Verification items for the finished model (mm, model axes). A direction names the side the tool comes from. Coordinates: 2 decimals unless noted, no trailing zeros. Order: outer loops, then holes, each group sorted by start corner. A loop starts at its lowest first (then second) coordinate and runs counter-clockwise, first axis right, second up. Notation, with made-up numbers: (52, 12) -> (57, 12) arc R14 cw to (57, 36) -> close; hole circle Ø1 at (51.25, -37). An arc over 180 degrees is marked (long way). Use CSV: the item, a comma, the result in double quotes. Start each with the question number.
1) Scan lines: line 1 along Y through (x, z) = (0, -1.9); line 2 along Y through (x, z) = (0, -0.8). Record each from-to range of solid material in increasing order.
2) Tool access check on faces 1 (the flat face through (8.6, 16.4, -0.508)), 2 (the flat face through (2.76, 1.57, 1.54)), 3 (the cylindrical face through (-0.33, -2.52, -1.77)). Record the directions out of +Z, -Z, +X, -X, +Y, -Y that give a thin tool (end or side, any length) a straight path to the whole face; none if there is none.
3) Sectioned sample at B-B on x = 0. Record the boundary of the cut face in (y, z) (3 decimals), then the cut area to 3 significant figures.
4) Release check for a two-part mould opening along X. For faces 4 (the cylindrical face through (0.201, 38.098, 1.377)), 5 (the flat face through (0.1, 3.556, -0.5)), 6 (the flat face through (2.737, -1.61, 1.542)), 7 (the flat face through (0, 15, 2.794)) record: released by +X, released by -X, zero draft, split by the parting line, or undercut.
5) Sectioned sample at A-A on z = 2.35. Record the boundary of the cut face in (x, y) (3 decimals).
6) Go/stop test with flat-tipped pins: pin 1 (0.8 mm diameter, centred on x = -9, y = 11.5, fed in from -Z); pin 2 (4.5 mm diameter, centred on x = 0, y = 0, fed in from +Z); pin 3 (1 mm diameter, centred on x = -2, y = 29, fed in from -Z). Record where each tip stops, or that it passes through.
7) Sectioned sample at C-C on y = 8. Record the boundary of the cut face in (x, z).
8) Sectioned sample at D-D on x = 4.25. Record the boundary of the cut face in (y, z).
from build123d import *

# Parameters (mm, degrees)
F0_W     = 1.016
F0_H     = 3.556
F0_H_2   = 5.588
F1_DEPTH = 2.794
F2_DEPTH = 0.508
F3_DEPTH = 1.016
F4_R     = 2.54
F5_DEPTH = 1.524
F6_R     = 1.397
F7_DEPTH = 5.334
F9_DEPTH = 2.54


with BuildPart() as f1:
    # F0 (on Top) → F1 (new body)
    with BuildSketch(Plane.XY):
        with BuildLine():
            Line((8.128, 28.956), (9.144, 28.956))
            ThreePointArc((9.144, 28.956), (0, 38.1), (-9.144, 28.956))
            Line((-9.144, 28.956), (-8.128, 28.956))
            Line((-8.128, 28.956), (-2.54, 28.956))
            ThreePointArc((-2.54, 28.956), (0, 31.496), (2.54, 28.956))
            Line((2.54, 28.956), (8.128, 28.956))
        make_face()
        with BuildLine():
            ThreePointArc((-8.128, 24.7669246844), (0, 19.812), (8.128, 24.7669246844))
            Line((8.128, 24.7669246844), (8.128, 28.956))
            Line((8.128, 28.956), (2.54, 28.956))
            ThreePointArc((2.54, 28.956), (0, 26.416), (-2.54, 28.956))
            Line((-2.54, 28.956), (-8.128, 28.956))
            Line((-8.128, 28.956), (-8.128, 24.7669246844))
        make_face()
        with BuildLine():
            Line((8.128, 24.7669246844), (8.128, 9.144))
            Line((8.128, 9.144), (9.144, 9.144))
            Line((9.144, 9.144), (9.144, 28.956))
            ThreePointArc((9.144, 28.956), (8.8863706877, 26.8007385309), (8.128, 24.7669246844))
        make_face()
        with BuildLine():
            Line((8.128, 28.956), (8.128, 24.7669246844))
            ThreePointArc((8.128, 24.7669246844), (8.8863706877, 26.8007385309), (9.144, 28.956))
            Line((9.144, 28.956), (8.128, 28.956))
        make_face()
        with BuildLine():
            ThreePointArc((-2.54, 28.956), (0, 26.416), (2.54, 28.956))
            Line((2.54, 28.956), (-2.54, 28.956))
        make_face()
        with BuildLine():
            Line((-2.54, 28.956), (2.54, 28.956))
            ThreePointArc((2.54, 28.956), (0, 31.496), (-2.54, 28.956))
        make_face()
        with BuildLine():
            ThreePointArc((-9.144, 28.956), (-8.8863706877, 26.8007385309), (-8.128, 24.7669246844))
            Line((-8.128, 24.7669246844), (-8.128, 28.956))
            Line((-8.128, 28.956), (-9.144, 28.956))
        make_face()
        with BuildLine():
            Line((-9.144, 9.144), (-8.128, 9.144))
            Line((-8.128, 9.144), (-8.128, 24.7669246844))
            ThreePointArc((-8.128, 24.7669246844), (-8.8863706877, 26.8007385309), (-9.144, 28.956))
            Line((-9.144, 28.956), (-9.144, 9.144))
        make_face()
        with BuildLine():
            Line((-8.128, 9.144), (8.128, 9.144))
            Line((8.128, 9.144), (8.128, 24.7669246844))
            ThreePointArc((8.128, 24.7669246844), (0, 19.812), (-8.128, 24.7669246844))
            Line((-8.128, 24.7669246844), (-8.128, 9.144))
        make_face()
        Polygon((-8.128, 3.556), (0, 3.556), (8.128, 3.556), (8.128, 9.144), (-8.128, 9.144), align=None)
        with BuildLine():
            ThreePointArc((-2.54, 0), (-1.7960512242, 1.7960512242), (0, 2.54))
            Line((0, 2.54), (0, 3.556))
            Line((0, 3.556), (-8.128, 3.556))
            Line((-8.128, 3.556), (-8.128, 0))
            Line((-8.128, 0), (-2.54, 0))
        make_face()
        with BuildLine():
            Line((0, -9.144), (0, -2.54))
            ThreePointArc((0, -2.54), (-1.7960512242, -1.7960512242), (-2.54, 0))
            Line((-2.54, 0), (-8.128, 0))
            Line((-8.128, 0), (-9.144, 0))
            Line((-9.144, 0), (-9.144, -9.144))
            Line((-9.144, -9.144), (0, -9.144))
        make_face()
        with Locations((-8.636, 1.778)):
            Rectangle(F0_W, F0_H)
        with BuildLine():
            ThreePointArc((0, 2.54), (1.7960512242, 1.7960512242), (2.54, 0))
            Line((2.54, 0), (8.128, 0))
            Line((8.128, 0), (8.128, 3.556))
            Line((8.128, 3.556), (0, 3.556))
            Line((0, 3.556), (0, 2.54))
        make_face()
        with Locations((8.636, 1.778)):
            Rectangle(F0_W, F0_H)
        with BuildLine():
            Line((8.128, 0), (2.54, 0))
            ThreePointArc((2.54, 0), (1.7960512242, -1.7960512242), (0, -2.54))
            Line((0, -2.54), (0, -9.144))
            Line((0, -9.144), (9.144, -9.144))
            Line((9.144, -9.144), (9.144, 0))
            Line((9.144, 0), (8.128, 0))
        make_face()
        with BuildLine():
            ThreePointArc((0, -2.54), (1.7960512242, -1.7960512242), (2.54, 0))
            Line((2.54, 0), (0, 0))
            Line((0, 0), (-2.54, 0))
            ThreePointArc((-2.54, 0), (-1.7960512242, -1.7960512242), (0, -2.54))
        make_face()
        with BuildLine():
            Line((0, 0), (2.54, 0))
            ThreePointArc((2.54, 0), (1.7960512242, 1.7960512242), (0, 2.54))
            ThreePointArc((0, 2.54), (-1.7960512242, 1.7960512242), (-2.54, 0))
            Line((-2.54, 0), (0, 0))
        make_face()
        with Locations((-8.636, 6.35)):
            Rectangle(F0_W, F0_H_2)
        with Locations((8.636, 6.35)):
            Rectangle(F0_W, F0_H_2)
    extrude(amount=F1_DEPTH)

    # F0 (on Top) → F2 (join)
    with BuildSketch(Plane.XY):
        with BuildLine():
            ThreePointArc((-9.144, 28.956), (-8.8863706877, 26.8007385309), (-8.128, 24.7669246844))
            Line((-8.128, 24.7669246844), (-8.128, 28.956))
            Line((-8.128, 28.956), (-9.144, 28.956))
        make_face()
        with BuildLine():
            Line((-9.144, 9.144), (-8.128, 9.144))
            Line((-8.128, 9.144), (-8.128, 24.7669246844))
            ThreePointArc((-8.128, 24.7669246844), (-8.8863706877, 26.8007385309), (-9.144, 28.956))
            Line((-9.144, 28.956), (-9.144, 9.144))
        make_face()
        with BuildLine():
            Line((8.128, 24.7669246844), (8.128, 9.144))
            Line((8.128, 9.144), (9.144, 9.144))
            Line((9.144, 9.144), (9.144, 28.956))
            ThreePointArc((9.144, 28.956), (8.8863706877, 26.8007385309), (8.128, 24.7669246844))
        make_face()
        with BuildLine():
            Line((8.128, 28.956), (8.128, 24.7669246844))
            ThreePointArc((8.128, 24.7669246844), (8.8863706877, 26.8007385309), (9.144, 28.956))
            Line((9.144, 28.956), (8.128, 28.956))
        make_face()
        with Locations((-8.636, 6.35)):
            Rectangle(F0_W, F0_H_2)
        with Locations((8.636, 6.35)):
            Rectangle(F0_W, F0_H_2)
    extrude(amount=-F2_DEPTH)

    # F0 (on Top) → F3 (join)
    with BuildSketch(Plane.XY):
        with BuildLine():
            Line((0, -9.144), (0, -2.54))
            ThreePointArc((0, -2.54), (-1.7960512242, -1.7960512242), (-2.54, 0))
            Line((-2.54, 0), (-8.128, 0))
            Line((-8.128, 0), (-9.144, 0))
            Line((-9.144, 0), (-9.144, -9.144))
            Line((-9.144, -9.144), (0, -9.144))
        make_face()
        with BuildLine():
            ThreePointArc((-2.54, 0), (-1.7960512242, 1.7960512242), (0, 2.54))
            Line((0, 2.54), (0, 3.556))
            Line((0, 3.556), (-8.128, 3.556))
            Line((-8.128, 3.556), (-8.128, 0))
            Line((-8.128, 0), (-2.54, 0))
        make_face()
        with BuildLine():
            ThreePointArc((0, -2.54), (1.7960512242, -1.7960512242), (2.54, 0))
            Line((2.54, 0), (0, 0))
            Line((0, 0), (-2.54, 0))
            ThreePointArc((-2.54, 0), (-1.7960512242, -1.7960512242), (0, -2.54))
        make_face()
        with BuildLine():
            Line((0, 0), (2.54, 0))
            ThreePointArc((2.54, 0), (1.7960512242, 1.7960512242), (0, 2.54))
            ThreePointArc((0, 2.54), (-1.7960512242, 1.7960512242), (-2.54, 0))
            Line((-2.54, 0), (0, 0))
        make_face()
        with BuildLine():
            ThreePointArc((0, 2.54), (1.7960512242, 1.7960512242), (2.54, 0))
            Line((2.54, 0), (8.128, 0))
            Line((8.128, 0), (8.128, 3.556))
            Line((8.128, 3.556), (0, 3.556))
            Line((0, 3.556), (0, 2.54))
        make_face()
        with BuildLine():
            Line((8.128, 0), (2.54, 0))
            ThreePointArc((2.54, 0), (1.7960512242, -1.7960512242), (0, -2.54))
            Line((0, -2.54), (0, -9.144))
            Line((0, -9.144), (9.144, -9.144))
            Line((9.144, -9.144), (9.144, 0))
            Line((9.144, 0), (8.128, 0))
        make_face()
        with Locations((-8.636, 1.778)):
            Rectangle(F0_W, F0_H)
        with Locations((8.636, 1.778)):
            Rectangle(F0_W, F0_H)
    extrude(amount=-F3_DEPTH)

    # F4 (on face) → F5 (join)
    with BuildSketch(Plane(origin=(0, 0, -1.016), x_dir=(1, 0, 0), z_dir=(0, 0, -1))):
        Circle(F4_R)
    extrude(amount=F5_DEPTH)

    # F6 (on face) → F7 (cut, through all)
    with BuildSketch(Plane(origin=(0, 0, -2.54), x_dir=(1, 0, 0), z_dir=(0, 0, -1))):
        Circle(F6_R)
    extrude(amount=-F7_DEPTH, mode=Mode.SUBTRACT)

    # F8 (on face) → F9 (cut)
    with BuildSketch(Plane.XY.offset(2.794)):
        Polygon((-1.8330871047, -3.175), (0, -3.175), (1.8330871047, -3.175), (3.6661742094, 0), (1.8330871047, 3.175), (-1.8330871047, 3.175), (-3.6661742094, 0), align=None)
        with BuildLine():
            ThreePointArc((1.397, 0), (0.9878281733, -0.9878281733), (0, -1.397))
            ThreePointArc((0, -1.397), (-0.9878281733, 0.9878281733), (1.397, 0))
        make_face(mode=Mode.SUBTRACT)
    extrude(amount=-F9_DEPTH, mode=Mode.SUBTRACT)


solid = f1.part
Answers follow:
1,line 1,"y = -2.54 to -1.4, 1.4 to 2.54"
1,line 2,"y = -9.14 to -1.4, 1.4 to 3.56"
2,face 1,"-Z, +X, -X, +Y"
2,face 2,"+Z"
2,face 3,"-Z"
3,outline,"(-9.144, -1.016) -> (-2.54, -1.016) -> (-2.54, -2.54) -> (-1.397, -2.54) -> (-1.397, 0.254) -> (-3.175, 0.254) -> (-3.175, 2.794) -> (-9.144, 2.794) -> close; (1.397, -2.54) -> (2.54, -2.54) -> (2.54, -1.016) -> (3.556, -1.016) -> (3.556, 0) -> (38.1, 0) -> (38.1, 2.794) -> (3.175, 2.794) -> (3.175, 0.254) -> (1.397, 0.254) -> close"
3,area,"129 mm²"
4,face 4,"split by the parting line"
4,face 5,"undercut"
4,face 6,"undercut"
4,face 7,"zero draft"
5,outline,"(-9.144, -9.144) -> (9.144, -9.144) -> (9.144, 28.956) arc R9.144 ccw to (-9.144, 28.956) -> close; hole (-3.666, 0) -> (-1.833, -3.175) -> (1.833, -3.175) -> (3.666, 0) -> (1.833, 3.175) -> (-1.833, 3.175) -> close"
6,pin 1,"stops at z = -0.51"
6,pin 2,"stops at z = 0.25"
6,pin 3,"stops at z = 0"
7,outline,"(-9.14, -0.51) -> (-8.13, -0.51) -> (-8.13, 0) -> (8.13, 0) -> (8.13, -0.51) -> (9.14, -0.51) -> (9.14, 2.79) -> (-9.14, 2.79) -> close"
8,outline,"(-9.14, -1.02) -> (3.56, -1.02) -> (3.56, 0) -> (37.05, 0) -> (37.05, 2.79) -> (-9.14, 2.79) -> close"
